Geometry: final body of the model. Coordinates: model frame, mm. A direction names the side the tool comes from. Give positions to 0.01 mm unless a question says otherwise; leave off trailing zeros. Write each loop counter-clockwise with the first axis right and the second up, starting at its lowest first coordinate (ties: lowest second). Pieces come first, ordered by that corner, then holes.
Autodesk Inventor part; units mm, degrees
ref_plane "YZ Plane" through (0, 0, 0) normal (1, 0, 0) x (0, 1, 0)
ref_plane "XZ Plane" through (0, 0, 0) normal (0, 1, 0) x (-1, 0, 0)
ref_plane "XY Plane" through (0, 0, 0) normal (0, 0, 1) x (1, 0, 0)
sketch "Sketch1" plane through (0, 0, 0) normal (0, 0, 1) x (1, 0, 0)
  circle A0 centre (-35.75, 35.75) radius 2.25
  circle A1 centre (35.75, 35.75) radius 2.25
  circle A2 centre (35.75, -35.75) radius 2.25
  circle A3 centre (-35.75, -35.75) radius 2.25
  line L0 (40, 40) -> (-40, 40)
  line L1 (-40, 40) -> (-40, -40)
  line L2 (-40, -40) -> (40, -40)
  line L3 (40, -40) -> (40, 40)
  circle A4 centre (0, 0) radius 35.75 construction
  line L4 (-35.75, 35.75) -> (35.75, -35.75) construction
  line L5 (-35.75, -35.75) -> (35.75, 35.75) construction
  line L6 (-24.5621, 25.9763) -> (-16.5896, 18.0038) construction
  line L7 (-25.9763, 24.5621) -> (16.5896, -18.0038) construction
  line L8 (24.5621, 25.9763) -> (18.5727, 19.987) construction
  line L9 (-24.5621, -25.9763) -> (16.9422, 15.528) construction
  line L10 (18.5727, 19.987) -> (17.1575, 18.5717) construction
  line L11 (17.1575, 18.5717) -> (16.5896, 18.0038) construction
  line L12 (0, 1.4142) -> (-18.0038, -16.5896) construction
  line L13 (0, 1.4142) -> (16.9422, -15.528) construction
  line L14 (16.5896, 18.0038) -> (15.528, 16.9422) construction
  line L15 (15.528, 16.9422) -> (0, 1.4142) construction
  arc A5 (16.9422, -15.528) -> (16.9422, 15.528) centre (0, 0) ccw
  line L16 (18.0038, 16.5896) -> (25.9763, 24.5621) construction
  line L17 (-16.5896, 18.0038) -> (0, 1.4142) construction
  arc A6 (-16.9422, 15.528) -> (-16.9422, -15.528) centre (0, 0) ccw
  arc A7 (-18.0038, 16.5896) -> (-18.0038, -16.5896) centre (0, 0) ccw
  line L18 (-18.0038, -16.5896) -> (-25.9763, -24.5621) construction
  arc A8 (-16.5896, -18.0038) -> (16.5896, -18.0038) centre (0, 0) ccw
  arc A9 (-15.528, -16.9422) -> (15.528, -16.9422) centre (0, 0) ccw
  line L19 (18.0038, -16.5896) -> (25.9763, -24.5621) construction
  line L20 (16.9422, -15.528) -> (18.0038, -16.5896) construction
  line L21 (16.9422, 15.528) -> (18.0038, 16.5896) construction
  arc A10 (15.528, 16.9422) -> (-15.528, 16.9422) centre (0, 0) ccw
  arc A11 (16.5896, 18.0038) -> (-16.5896, 18.0038) centre (0, 0) ccw
  line L22 (16.5896, -18.0038) -> (24.5621, -25.9763) construction
  arc A12 (18.0038, -16.5896) -> (18.0038, 16.5896) centre (0, 0) ccw
  arc A13 (24.5621, 25.9763) -> (-24.5621, 25.9763) centre (0, 0) ccw
  arc A14 (25.9763, -24.5621) -> (25.9763, 24.5621) centre (0, 0) ccw
  arc A15 (-24.5621, -25.9763) -> (24.5621, -25.9763) centre (0, 0) ccw
  arc A16 (-25.9763, 24.5621) -> (-25.9763, -24.5621) centre (0, 0) ccw
  line L23 (-16.5896, 18.0038) -> (-24.5621, 25.9763)
  line L24 (-18.0038, 16.5896) -> (-25.9763, 24.5621)
  line L25 (16.5896, 18.0038) -> (24.5621, 25.9763)
  line L26 (25.9763, 24.5621) -> (18.0038, 16.5896)
  line L27 (18.0038, -16.5896) -> (25.9763, -24.5621)
  line L28 (24.5621, -25.9763) -> (16.5896, -18.0038)
  line L29 (-24.5621, -25.9763) -> (-16.5896, -18.0038)
  line L30 (-18.0038, -16.5896) -> (-25.9763, -24.5621)
  line L31 (-16.9422, -15.528) -> (-1.4142, 0)
  line L32 (-15.528, -16.9422) -> (0, -1.4142)
  line L33 (-1.4142, 0) -> (-16.9422, 15.528)
  line L34 (-15.528, 16.9422) -> (0, 1.4142)
  line L35 (0, -1.4142) -> (15.528, -16.9422)
  line L36 (16.9422, -15.528) -> (1.4142, 0)
  line L37 (1.4142, 0) -> (16.9422, 15.528)
  line L38 (15.528, 16.9422) -> (0, 1.4142)
  dimension "d8" = 2
  dimension "d9" = 1
extrude "Extrusion3" add sketch "Sketch1" along normal blind 1.5
fillet "Fillet3" radius 4 4 edges at (-40, -40, 0.75) (40, -40, 0.75) (40, 40, 0.75) (-40, 40, 0.75)
properties part number "grid"
Q1. Section D-D on z = 0.8. Count the separate pieces of the cut face and the enclosed holes in it, plus the area to 3 significant figures.
Filled sheet:
separate pieces: 1
enclosed holes: 12
area: 2,800 mm2
Q2. Pin query (flat end, axial travel): P1, Ø6, axis at x = 35.75, y = -35.75, coming from the -Z side. Return the tip coordinate at first contact, or that it passes through.
Filled sheet:
P1: stops at z = 0
Q3. Ray query, line 1 along Y through (x, z) = (13.5, 0.1); line 2 along X through (y, z) = (-17, 0.45); line 3 along Y through (x, z) = (-8, 1). Return the intervals inside material, ascending.
Filled sheet:
line 1: y = -40 to -33.1, -20.42 to -18.6, -14.91 to -12.09, 12.09 to 14.91, 18.6 to 20.42, 33.1 to 40
line 2: x = -40 to -31.45, -18.41 to -15.46, 15.46 to 18.41, 31.45 to 40
line 3: y = -40 to -34.84, -23.14 to -21.54, -9.41 to -6.59, 6.59 to 9.41, 21.54 to 23.14, 34.84 to 40
Q4. Section A-A on x = 29.5. Output: boundary loops of the cut face in (y, z).
Filled sheet:
outline: (-40, 0) - (-20.19, 0) - (-20.19, 1.5) - (-40, 1.5) - close; (20.19, 0) - (40, 0) - (40, 1.5) - (20.19, 1.5) - close
Q5. Section B-B on y = -21.5. Output: boundary loops of the cut face in (x, z).
Filled sheet:
outline: (-40, 0) - (-28.56, 0) - (-28.56, 1.5) - (-40, 1.5) - close; (-22.91, 0) - (-20.09, 0) - (-20.09, 1.5) - (-22.91, 1.5) - close; (-11.71, 0) - (-8.12, 0) - (-8.12, 1.5) - (-11.71, 1.5) - close; (8.12, 0) - (11.71, 0) - (11.71, 1.5) - (8.12, 1.5) - close; (20.09, 0) - (22.91, 0) - (22.91, 1.5) - (20.09, 1.5) - close; (28.56, 0) - (40, 0) - (40, 1.5) - (28.56, 1.5) - close
Q6. Pull-direction query (X, two-part tool) for faces 3 (the cylindrical face through (-38.859, -38.797, 0.76)), 4 (the flat face through (-7.873, -9.287, 0.74)), 5 (the flat face through (-7.873, 9.287, 0.74)), 6 (the cylindrical face through (38.859, 38.797, 0.76)); classes: released by +X, released by -X, zero draft, split by the parting line, or undercut.
Filled sheet:
face 3: released by -X
face 4: undercut
face 5: undercut
face 6: released by +X
Q7. Access query for faces 1 (the cylindrical face through (24.48, 0.26, 0.74)), 2 (the cylindrical face through (38.797, -38.859, 0.76)). Directions: +Z, -Z, +X, -X, +Y, -Y. A direction counts if a zero-diameter tool reaches every point of the face in a straight line with its end or side. Return the directions, or none.
Filled sheet:
face 1: +Z, -Z
face 2: +Z, -Z, +X, -Y
Q8. Section C-C on x = -3. Output: boundary loops of the cut face in (y, z), plus the area to 3 significant figures.
Filled sheet:
outline: (-40, 0) - (-35.62, 0) - (-35.62, 1.5) - (-40, 1.5) - close; (-24.3, 0) - (-22.79, 0) - (-22.79, 1.5) - (-24.3, 1.5) - close; (-4.41, 0) - (-1.59, 0) - (-1.59, 1.5) - (-4.41, 1.5) - close; (1.59, 0) - (4.41, 0) - (4.41, 1.5) - (1.59, 1.5) - close; (22.79, 0) - (24.3, 0) - (24.3, 1.5) - (22.79, 1.5) - close; (35.62, 0) - (40, 0) - (40, 1.5) - (35.62, 1.5) - close
area: 26.1 mm2
